Autodesk Inventor part; units mm, degrees
ref_plane "YZ Plane" through (0, 0, 0) normal (1, 0, 0) x (0, 1, 0)
ref_plane "XZ Plane" through (0, 0, 0) normal (0, 1, 0) x (-1, 0, 0)
ref_plane "XY Plane" through (0, 0, 0) normal (0, 0, 1) x (1, 0, 0)
sketch "Sketch1" plane through (0, 0, 0) normal (0, 0, 1) x (1, 0, 0)
  circle A0 centre (0, 0) radius 10
  dimension "d0" = 20
extrude "Extrusion1" add sketch "Sketch1" along normal blind 4.5
sketch "Sketch2" plane through (0, 0, 4.5) normal (0, 0, 1) x (1, 0, 0)
  circle A0 centre (0, 0) radius 10
  line L0 (-6, -8) -> (6, -8)
  line L1 (6, -8) -> (6, 8)
  line L2 (6, 8) -> (-6, 8)
  line L3 (-6, 8) -> (-6, -8)
  line L4 (-6, -8) -> (6, 8) construction
  line L5 (6, -8) -> (-6, 8) construction
  arc A1 (6, 8) -> (-6, 8) centre (0, 0) ccw
  arc A2 (-6, -8) -> (6, -8) centre (0, 0) ccw
  dimension "d3" = 12
extrude "Extrusion2" add sketch "Sketch2" along normal blind 10 contours L2 A0 | L1 L0 L3 L2 | A0 L0
sketch "Sketch3" plane through (0, 0, 0) normal (0, 0, -1) x (-1, 0, 0)
  circle A0 centre (0, 0) radius 11.5
  dimension "d6" = 23
extrude "Extrusion3" add sketch "Sketch3" along normal blind 1
fillet "Fillet1" radius 2 1 edges at (11.5, 0, -1)
sketch "Sketch4" plane through (0, 0, 14.5) normal (0, 0, 1) x (1, 0, 0)
  circle A0 centre (0, 6.6483) radius 2.5
  circle A1 centre (0, 0) radius 2.5
  circle A2 centre (0, -6.4728) radius 2.5
  dimension "d10" = 5
  dimension "d11" = 5
  dimension "d12" = 5
extrude "Extrusion4" add sketch "Sketch4" along normal blind 10
properties part number "Switch_DC_Pilot"
Model file for the job. Use its own axes, mm. A direction names the side the tool comes from. Give positions to 0.01 mm unless a question says otherwise; leave off trailing zeros. Write each loop counter-clockwise with the first axis right and the second up, starting at its lowest first coordinate (ties: lowest second). Pieces come first, ordered by that corner, then holes. Notation, with made-up numbers: M -18,-31.5 L 16,-31.5 A14 ccw 16,-25.5 Z; hole C 82,5 d2. An arc over 180 degrees is marked long. Use a Markdown table: item, result.
1) Pull direction Y, two halves, no side cores. Call faces 5 (the cylindrical face through (9.54, -3, 3.93)), 6 (the flat face through (0, 0, -1)), 7 (the cylindrical face through (-0.33, -8.95, 19.43)): +Y half, -Y half, draft (parallel to the pull), parting line (faces both ways), or undercut.
Responses:
| item | result |
|---|---|
| face 5 | parting line |
| face 6 | draft |
| face 7 | undercut |
2) Drill centre lines: line 1 (Y direction, x = -1, z = 17); line 2 (X direction, y = -4.5, z = 6); line 3 (Z direction, x = 9, y = -1.25). Where is each one in solid material? Low to high. Write a range as from..to.
Responses:
| item | result |
|---|---|
| line 1 | y = -8.76..-4.18, -2.29..2.29, 4.36..8.94 |
| line 2 | x = -6..6 |
| line 3 | z = -1..4.5 |
3) Cut at C-C (z = 18.25). List the corners of the cut face in (x, y), and give its area (3 significant figures).
Responses:
| item | result |
|---|---|
| outline | C 0,-6.47 d5; C 0,0 d5; C 0,6.65 d5 |
| area | 58.9 mm2 |
4) Tool access for faces 1 (the flat face through (8, 0, 4.5)), 2 (the flat face through (-6, 0, 9)), 3 (the flat face through (0, -6, 24.5)), 4 (the cylindrical face through (-0.54, 2.44, 19.43)): list every direction of +Z, -Z, +X, -X, +Y, -Y with a clear straight run to the whole face (end or side of a thin tool).
Responses:
| item | result |
|---|---|
| face 1 | +Z, +X, +Y, -Y |
| face 2 | +Z, -X, +Y, -Y |
| face 3 | +Z, +X, -X, +Y, -Y |
| face 4 | +Z |
5) Pin check, flat tips, straight feed: pin 1 (8 mm diameter, centred on y = 1, z = 16.5, fed in from -X); pin 2 (8 mm diameter, centred on x = -9, y = 6.5, fed in from +Z); pin 3 (8 mm diameter, centred on y = 0, z = 8, fed in from -X). Stop position of each tip, or through.
Responses:
| item | result |
|---|---|
| pin 1 | stops at x = -6 |
| pin 2 | stops at z = 14.5 |
| pin 3 | stops at x = -10 |
6) Cut at A-A (y = 0). List the corners of the cut face in (x, z), and give its area (3 significant figures).
Responses:
| item | result |
|---|---|
| outline | M -11.5,0 A2 ccw -9.77,-1 L 9.77,-1 A2 ccw 11.5,0 L 10,0 L 10,4.5 L 6,4.5 L 6,14.5 L 2.5,14.5 L 2.5,24.5 L -2.5,24.5 L -2.5,14.5 L -6,14.5 L -6,4.5 L -10,4.5 L -10,0 Z |
| area | 282 mm2 |
7) Cut at D-D (z = 3.5). List the corners of the cut face in (x, y).
Responses:
| item | result |
|---|---|
| outline | C 0,0 d20 |
8) Cut at B-B (x = 0). List the corners of the cut face in (y, z).
Responses:
| item | result |
|---|---|
| outline | M -11.5,0 A2 ccw -9.77,-1 L 9.77,-1 A2 ccw 11.5,0 L 10,0 L 10,14.5 L 9.15,14.5 L 9.15,24.5 L 4.15,24.5 L 4.15,14.5 L 2.5,14.5 L 2.5,24.5 L -2.5,24.5 L -2.5,14.5 L -3.97,14.5 L -3.97,24.5 L -8.97,24.5 L -8.97,14.5 L -10,14.5 L -10,0 Z |
